Verification items for the finished model (mm, model axes). Give positions to 0.01 mm unless a question says otherwise; leave off trailing zeros. Order: outer loops, then holes, each group sorted by start corner. A loop starts at its lowest first (then second) coordinate and runs counter-clockwise, first axis right, second up. Notation, with made-up numbers: M 7.5,44 L 53.5,44 A10 cw 53.5,50 Z; hole C 21,75 d7. An arc over 180 degrees is marked long. Answer as a JSON object with one key per item and string values.
Autodesk Inventor part; units mm, degrees
ref_plane "YZ Plane" through (0, 0, 0) normal (1, 0, 0) x (0, 1, 0)
ref_plane "XZ Plane" through (0, 0, 0) normal (0, 1, 0) x (-1, 0, 0)
ref_plane "XY Plane" through (0, 0, 0) normal (0, 0, 1) x (1, 0, 0)
sketch "Sketch1" plane through (0, 0, 0) normal (1, 0, 0) x (0, 1, 0)
  circle A0 centre (-42.0801, -52.5105) radius 133.35
  dimension "d38" = 266.7
extrude "Extrusion1" add sketch "Sketch1" along normal blind 5.08
fillet "Fillet1" radius 2.286 1 edges at (5.08, -175.4301, -52.5105)
sketch "Sketch2" plane through (5.08, -42.0801, -52.5105) normal (1, 0, 0) x (0, 0, -1)
  line L0 (0.865, -2.45) -> (-0.865, -2.45)
  line L1 (-1.5, -1.815) -> (-1.5, 1.815)
  line L2 (-0.865, 2.45) -> (0.865, 2.45)
  line L3 (1.5, 1.815) -> (1.5, -1.815)
  line L4 (1.5, -2.45) -> (-1.5, 2.45) construction
  line L5 (-1.5, -2.45) -> (1.5, 2.45) construction
  arc A0 (-0.865, 2.45) -> (-1.5, 1.815) centre (-0.865, 1.815) ccw
  arc A1 (1.5, 1.815) -> (0.865, 2.45) centre (0.865, 1.815) ccw
  arc A2 (-1.5, -1.815) -> (-0.865, -2.45) centre (-0.865, -1.815) ccw
  arc A3 (0.865, -2.45) -> (1.5, -1.815) centre (0.865, -1.815) ccw
  point P0 (-52.5105, 42.0801)
  point P1 (0, 0)
extrude "Extrusion3" cut sketch "Sketch2" against normal blind 5.08
sketch "Sketch4" plane through (5.08, -42.0801, -52.5105) normal (1, 0, 0) x (0, 0, -1)
  circle A0 centre (-63.4701, -44.45) radius 1.27
  circle A1 centre (-63.5, 50.8) radius 1.27
  circle A2 centre (69.85, 50.8239) radius 1.27
  circle A3 centre (69.8799, -44.4261) radius 1.27
  point P0 (-52.5105, 42.0801)
extrude "Extrusion5" cut sketch "Sketch4" against normal through all
properties part number "Rotating Base"
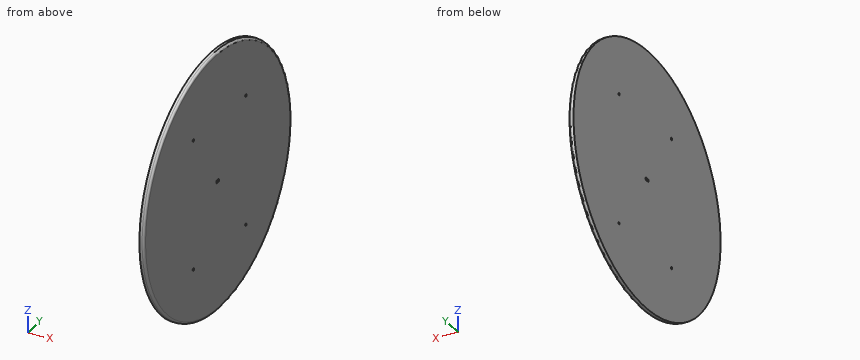
Q1. Material ranges on L1, parallel to Z at x = 3.75, y = -85.5; L2, parallel to X at y = 60, z = -135.5; L3, parallel to Z at x = 4.3, y = -86, recorded low to high.
Resolved:
{"L1": "z = -178.37 to -123.17, -121.62 to 10.22, 11.7 to 73.35", "L2": "x = 0 to 5.03", "L3": "z = -177.82 to -123.56, -121.23 to 9.81, 12.11 to 72.8"}
Q2. Section check A-A on x = 3.8. Record the cut outline in (y, z) (1 decimal).
Resolved:
{"outline": "C -42.1,-52.5 d266.2; hole C -86.5,-122.4 d2.5; hole C -86.5,11 d2.5; hole M -44.5,-53.4 A0.6 ccw -43.9,-54 L -40.3,-54 A0.6 ccw -39.6,-53.4 L -39.6,-51.6 A0.6 ccw -40.3,-51 L -43.9,-51 A0.6 ccw -44.5,-51.6 Z; hole C 8.7,11 d2.5; hole C 8.7,-122.4 d2.5"}
Q3. Gauge pin test, flat ends, axial feed: pin 1 Ø4 at (y, z) = (8.72, 10.99) entering from -X; pin 2 Ø3 at (x, z) = (2.5, -154.5) entering from -Y; pin 3 Ø2 at (y, z) = (-86.51, -122.39) entering from -X; pin 4 Ø2 at (x, y) = (2.5, -34) entering from -Z. Record the tip position at first contact, or that the pin passes through.
Resolved:
{"pin 1": "stops at x = 0", "pin 2": "stops at y = -129.74", "pin 3": "passes through", "pin 4": "stops at z = -185.67"}
